Can you work these out from the model? Positions are in its coordinate system, mm. Face numbers are marked on the shaded views. Coordinates: 2 decimals unless noted, no trailing zeros. Write each loop counter-clockwise with the first axis right and the second up, starting at its lowest first coordinate (ties: lowest second). Pieces come first, ordered by that corner, then holes. Notation, with made-up numbers: (0, -39) -> (29, -39) arc R27 cw to (29, -13) -> close; hole circle Ø5 at (44.5, -35). An arc over 180 degrees is marked (long way). Answer as CSV lines item,"result". Start each with the question number.
```python
from build123d import *

# Parameters (mm, degrees)
SKETCH1_W           = 15
SKETCH1_H           = 15
SKETCH1_R           = 2.1
BOSS_EXTRUDE1_DEPTH = 8
SKETCH2_R           = 2.5
CUT_EXTRUDE1_DEPTH  = 16
SKETCH3_R           = 1.05
CUT_EXTRUDE2_DEPTH  = 16


with BuildPart() as part:
    # Sketch1 → Boss-Extrude1 (new body)
    with BuildSketch(Plane.XY):
        with Locations((4.5, -3.5)):
            Rectangle(SKETCH1_W, SKETCH1_H)
        Circle(SKETCH1_R, mode=Mode.SUBTRACT)
    extrude(amount=BOSS_EXTRUDE1_DEPTH)

    # Sketch2 → Cut-Extrude1 (cut, through all)
    with BuildSketch(Plane.XZ.offset(11)):
        with Locations((7, 4)):
            Circle(SKETCH2_R)
    extrude(amount=-CUT_EXTRUDE1_DEPTH, mode=Mode.SUBTRACT)

    # Sketch3 → Cut-Extrude2 (cut, through all)
    with BuildSketch(Plane.XZ.offset(11)):
        with Locations((3.6, 2)):
            Circle(SKETCH3_R)
    extrude(amount=-CUT_EXTRUDE2_DEPTH, mode=Mode.SUBTRACT)


solid = part.part
```
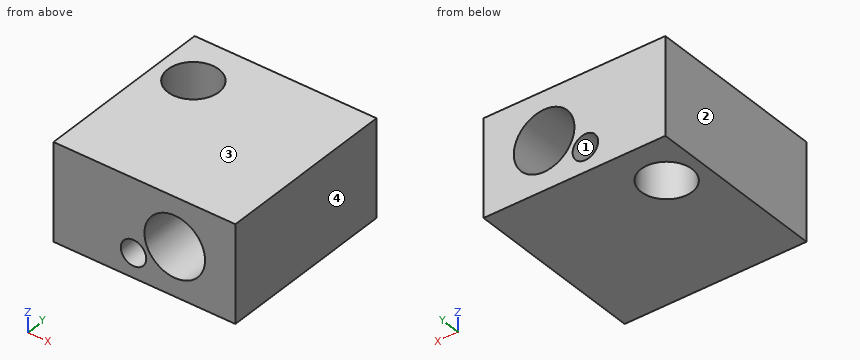
Q1. Imagine slicing it at C-C (x = 3.6). Write out the boundary of the cut face in (y, z).
Q2. Imagine slicing it at A-A (y = 0). Write out the boundary of the cut face in (x, z), then the cut area to 3 significant figures.
Q3. If we mould it in two halves opening along X, with no side actions, what happens to the marked faces 1, 2, 3 and 4? For each: released by +X, released by -X, zero draft, split by the parting line, or undercut.
Q4. Imagine slicing it at D-D (z = 2). Write out the boundary of the cut face in (x, y), then the cut area to 3 significant figures.
Q5. Imagine slicing it at B-B (z = 4). Write out the boundary of the cut face in (x, y), then the cut area to 3 significant figures.
Q6. I need wall thicknesses on L1, parallel to Z at x = 3.6, y = -1.5; L2, parallel to X at y = 1, z = 5.25; L3, parallel to Z at x = 7, y = -4.75. Which ranges of each line are inside material? Lowest first, please.
Entries:
1,outline,"(-11, 0) -> (4, 0) -> (4, 0.95) -> (-11, 0.95) -> close; (-11, 3.05) -> (4, 3.05) -> (4, 8) -> (-11, 8) -> close"
2,outline,"(-3, 0) -> (-2.1, 0) -> (-2.1, 8) -> (-3, 8) -> close; (2.1, 0) -> (12, 0) -> (12, 8) -> (2.1, 8) -> close; hole circle Ø2.1 at (3.6, 2); hole circle Ø5 at (7, 4)"
2,area,"63.3 mm2"
3,face 1,"undercut"
3,face 2,"released by -X"
3,face 3,"zero draft"
3,face 4,"released by +X"
4,outline,"(-3, -11) -> (2.55, -11) -> (2.55, 4) -> (-3, 4) -> close; (4.65, -11) -> (5.5, -11) -> (5.5, 4) -> (4.65, 4) -> close; (8.5, -11) -> (12, -11) -> (12, 4) -> (8.5, 4) -> close; hole circle Ø4.2 at (0, 0)"
4,area,"135 mm2"
5,outline,"(-3, -11) -> (4.5, -11) -> (4.5, 4) -> (-3, 4) -> close; (9.5, -11) -> (12, -11) -> (12, 4) -> (9.5, 4) -> close; hole circle Ø4.2 at (0, 0)"
5,area,"136 mm2"
6,L1,"0 to 0.95, 3.05 to 8"
6,L2,"-3 to -1.85, 1.85 to 4.83, 9.17 to 12"
6,L3,"0 to 1.5, 6.5 to 8"
